```python
from build123d import *

# Parameters (mm, degrees)
SKETCH5_W           = 30
SKETCH5_H           = 29.75
SKETCH5_R           = 2.5
SKETCH5_R_2         = 1
BOSS_EXTRUDE3_DEPTH = 5
SKETCH10_R          = 2
CUT_EXTRUDE8_DEPTH  = 2.5
SKETCH11_W          = 30
SKETCH11_H          = 10.75
BOSS_EXTRUDE4_DEPTH = 56
BOSS_EXTRUDE5_DEPTH = 5
SKETCH13_R          = 6.25
CUT_EXTRUDE9_DEPTH  = 1.5
SKETCH16_R          = 3.5
CUT_EXTRUDE10_DEPTH = 4.25
SKETCH17_R          = 2
CUT_EXTRUDE11_DEPTH = 6.5


with BuildPart() as part:
    # Sketch5 → Boss-Extrude3 (new body)
    with BuildSketch(Plane(origin=(0, 0, 0), x_dir=(0, 0, -1), z_dir=(1, 0, 0))):
        with Locations((0, -5.375)):
            Rectangle(SKETCH5_W, SKETCH5_H)
        Circle(SKETCH5_R, mode=Mode.SUBTRACT)
        with Locations((6.495190528, 3.75)):
            Circle(SKETCH5_R_2, mode=Mode.SUBTRACT)
        with Locations((0, -7.5)):
            Circle(SKETCH5_R_2, mode=Mode.SUBTRACT)
        with Locations((-6.495190528, 3.75)):
            Circle(SKETCH5_R_2, mode=Mode.SUBTRACT)
    extrude(amount=-BOSS_EXTRUDE3_DEPTH)

    # Sketch10 → Cut-Extrude8 (cut)
    with BuildSketch(Plane(origin=(0, 0, 0), x_dir=(0, 0, -1), z_dir=(1, 0, 0))):
        with Locations((-6.495190528, 3.75)):
            Circle(SKETCH10_R)
        with Locations((6.495190528, 3.75)):
            Circle(SKETCH10_R)
        with Locations((0, -7.5)):
            Circle(SKETCH10_R)
    extrude(amount=-CUT_EXTRUDE8_DEPTH, mode=Mode.SUBTRACT)

    # Sketch11 → Boss-Extrude4 (add)
    with BuildSketch(Plane.ZY.offset(5)):
        with Locations((0, -14.875)):
            Rectangle(SKETCH11_W, SKETCH11_H)
    extrude(amount=BOSS_EXTRUDE4_DEPTH)

    # Sketch12 → Boss-Extrude5 (add)
    with BuildSketch(Plane(origin=(0, 0, -15), x_dir=(-1, 0, 0), z_dir=(0, 0, -1))):
        Polygon((5, -9.5), (61, -9.5), (5, 9.5), align=None)
    boss_extrude5 = extrude(amount=-BOSS_EXTRUDE5_DEPTH)

    # Mirror1: Boss-Extrude5 across plane
    add(boss_extrude5.mirror(Plane.XY))

    # Sketch13 → Cut-Extrude9 (cut)
    with BuildSketch(Plane.ZY.offset(5)):
        Circle(SKETCH13_R)
    extrude(amount=-CUT_EXTRUDE9_DEPTH, mode=Mode.SUBTRACT)

    # Sketch16 → Cut-Extrude10 (cut)
    with BuildSketch(Plane(origin=(0, -9.5, 0), x_dir=(1, 0, 0), z_dir=(0, 1, 0))):
        with Locations(Location((-11, 6.5, 0), (0, 0, 270))):
            Circle(SKETCH16_R)
        with Locations(Location((-56, 6.5, 0), (0, 0, 270))):
            Circle(SKETCH16_R)
        with Locations(Location((-56, -6.5, 0), (0, 0, 270))):
            Circle(SKETCH16_R)
        with Locations(Location((-11, -6.5, 0), (0, 0, 270))):
            Circle(SKETCH16_R)
    extrude(amount=-CUT_EXTRUDE10_DEPTH, mode=Mode.SUBTRACT)

    # Sketch17 → Cut-Extrude11 (cut)
    with BuildSketch(Plane(origin=(0, -13.75, 0), x_dir=(1, 0, 0), z_dir=(0, 1, 0))):
        with Locations(Location((-56, 6.5, 0), (0, 0, 270))):
            Circle(SKETCH17_R)
        with Locations(Location((-11, 6.5, 0), (0, 0, 270))):
            Circle(SKETCH17_R)
        with Locations(Location((-11, -6.5, 0), (0, 0, 270))):
            Circle(SKETCH17_R)
        with Locations(Location((-56, -6.5, 0), (0, 0, 270))):
            Circle(SKETCH17_R)
    extrude(amount=-CUT_EXTRUDE11_DEPTH, mode=Mode.SUBTRACT)


solid = part.part
```
Design review of the part built by this model. Coordinates are the model's own, in mm. A direction names the side the tool comes from. Round coordinates to 2 decimals unless told otherwise and drop trailing zeros. Write each loop counter-clockwise with the first axis right and the second up, starting at its lowest first coordinate (ties: lowest second). Pieces come first, ordered by that corner, then holes. Notation, with made-up numbers: (33.25, 46.25) -> (50.25, 46.25) arc R9 ccw to (50.25, 57.25) -> close; hole circle Ø5 at (41, -18.5). An arc over 180 degrees is marked (long way). Answer in a Markdown table with one row per item.
Q1. Clearance check with flat-ended pins moving along their axes: pin 1 Ø2 at (x, z) = (-47, 6.5) entering from +Y; pin 2 Ø16 at (y, z) = (0, 0) entering from -X; pin 3 Ø6.5 at (x, z) = (-11, 6.5) entering from +Y. State where each tip first meets the part, or that it passes through.
The answers:
| item | result |
|---|---|
| pin 1 | y = -9.5 |
| pin 2 | x = -5 |
| pin 3 | y = -13.75 |
Q2. Take a section at B-B, the plane y = -11.5. State the section outline as (x, z) points, then the cut area to 3 significant figures.
The answers:
| item | result |
|---|---|
| outline | (-61, -15) -> (0, -15) -> (0, 15) -> (-61, 15) -> close; hole circle Ø7 at (-56, -6.5); hole circle Ø7 at (-56, 6.5); hole circle Ø7 at (-11, -6.5); hole circle Ø7 at (-11, 6.5) |
| area | 1,680 mm² |
Q3. Take a section at A-A, the plane y = 0. State the section outline as (x, z) points.
The answers:
| item | result |
|---|---|
| outline | (-33, -15) -> (0, -15) -> (0, -2.5) -> (-3.5, -2.5) -> (-3.5, -6.25) -> (-5, -6.25) -> (-5, -10) -> (-33, -10) -> close; (-33, 10) -> (-5, 10) -> (-5, 6.25) -> (-3.5, 6.25) -> (-3.5, 2.5) -> (0, 2.5) -> (0, 15) -> (-33, 15) -> close |
Q4. For faces 1 (the face through (-20, -4, 10)), 2 (the face through (-33, 0, 13)), 3 (the face through (-58, -13.75, 8)), list the 3-axis set-ups (+Z, -Z, +X, -X, +Y, -Y) from which the entire face can be reached by the end or side of a thin tool; tool diameter is ignored.
The answers:
| item | result |
|---|---|
| face 1 | -X, +Y |
| face 2 | +Z, -Z, -X, +Y |
| face 3 | +Y |
Q5. Take a section at D-D, the plane z = -13. State the section outline as (x, y) points, then the cut area to 3 significant figures.
The answers:
| item | result |
|---|---|
| outline | (-61, -20.25) -> (0, -20.25) -> (0, 9.5) -> (-5, 9.5) -> (-61, -9.5) -> close |
| area | 1,280 mm² |
Q6. To check wall thickness, follow L1, parallel to X at y = -10.8, z = 6.5; L2, parallel to X at y = -17, z = -6.5; L3, parallel to Z at x = -6.5, y = 4.75. State the ranges of each line that lie inside material, in increasing order. Write a range as [from, to].
The answers:
| item | result |
|---|---|
| L1 | [-61, -59.5], [-52.5, -14.5], [-7.5, 0] |
| L2 | [-61, -58], [-54, -13], [-9, 0] |
| L3 | [-15, -10], [10, 15] |
Q7. Take a section at C-C, the plane x = -17. State the section outline as (y, z) points, then the cut area to 3 significant figures.
The answers:
| item | result |
|---|---|
| outline | (-20.25, -15) -> (5.43, -15) -> (5.43, -10) -> (-9.5, -10) -> (-9.5, 10) -> (5.43, 10) -> (5.43, 15) -> (-20.25, 15) -> close |
| area | 472 mm² |
Q8. Draft analysis for pull direction Y (two halves, no side actions). For faces 4 (the face through (-54.017, -16.954, -6.76)), 5 (the face through (-58, -13.75, -5)), 6 (the face through (-1.23, 2.53, 8.08)), state which applies: +Y half, -Y half, draft (parallel to the pull), parting line (faces both ways), or undercut.
The answers:
| item | result |
|---|---|
| face 4 | draft |
| face 5 | +Y half |
| face 6 | undercut |
